Source: CAD feature listing. Evaluate the final solid. Frame: model axes, mm. Face numbers are marked on the shaded views. A direction names the side the tool comes from. Give positions to 0.01 mm unless a question says otherwise; leave off trailing zeros. Order: outer loops, then holes, each group sorted by start corner. A loop starts at its lowest first (then second) coordinate and runs counter-clockwise, first axis right, second up. Notation, with made-up numbers: M 74.5,33 L 114.5,33 A20 cw 114.5,51 Z; hole C -8,59.25 d11. An arc over 180 degrees is marked long. Use CSV: the item, a comma, the result in double quotes. Start each with the question number.
1. Section query C-C, the plane z = 0. Return the cut outline in (x, y).
2. Section query D-D, the plane x = 27. Return the cut outline in (y, z), plus the area to 3 significant figures.
3. Line query: line 1 along Z through (x, y) = (40.5, 3.55); line 2 along Z through (x, y) = (38, 4.5); line 3 along X through (y, z) = (1.75, -10). Output: solid intervals per line, ascending. Write a range as [from, to].
4. Section query A-A, the plane y = 2.7. Return the cut outline in (x, z), plus the area to 3 significant figures.
5. Pin query (flat end, axial travel): P1, Ø1.5, axis at x = 35, y = 5, coming from the -Z side; P2, Ø0.5, axis at y = 5.5, z = -7, coming from the +X side; P3, Ø10, axis at x = 12, z = -2, coming from the -Y side. Return the tip coordinate at first contact, or that it passes through.
6. Section query B-B, the plane x = 40.5. Return the cut outline in (y, z).
7. Mould query, pull axis X, two halves, no side actions, for the marked faces 1, 2, 3 and 4. Classes: released by +X, released by -X, zero draft, split by the parting line, or undercut.
8. Reachability of the marked faces 5, 6 and 7 from +Z, -Z, +X, -X, +Y, -Y: full face, straight path, thin tool, end or side. Return the list, or none.
from build123d import *

# Parameters (mm, degrees)
CROQUIS1_R              = 2.25
SALIENTE_EXTRUIR2_DEPTH = 6
CROQUIS2_W              = 8
CROQUIS2_H              = 30
CORTAR_EXTRUIR1_DEPTH   = 1


with BuildPart() as part:
    # Croquis1 → Saliente-Extruir2 (new body)
    with BuildSketch(Plane(origin=(0, 0, 0), x_dir=(1, 0, 0), z_dir=(0, 1, 0))):
        with BuildLine():
            Line((1, 20), (25.839745962, 20))
            Line((25.839745962, 20), (34.5, 15))
            Line((34.5, 15), (44.5, 15))
            Line((44.5, 15), (44.5, -15))
            Line((44.5, -15), (34.5, -15))
            Line((34.5, -15), (25.839745962, -20))
            Line((25.839745962, -20), (1, -20))
            Line((1, -20), (1, -16.720122607))
            ThreePointArc((1, -16.720122607), (16.75, 0), (1, 16.720122607))
            Line((1, 16.720122607), (1, 20))
        make_face()
        with Locations(Location((40.5, 10, 0), (0, 0, 270))):
            Circle(CROQUIS1_R, mode=Mode.SUBTRACT)
        with Locations(Location((40.5, -10, 0), (0, 0, 270))):
            Circle(CROQUIS1_R, mode=Mode.SUBTRACT)
    extrude(amount=SALIENTE_EXTRUIR2_DEPTH)

    # Croquis2 → Cortar-Extruir1 (cut)
    with BuildSketch(Plane(origin=(0, 6, 0), x_dir=(1, 0, 0), z_dir=(0, 1, 0))):
        with Locations((40.5, 0)):
            Rectangle(CROQUIS2_W, CROQUIS2_H)
    extrude(amount=-CORTAR_EXTRUIR1_DEPTH, mode=Mode.SUBTRACT)

    # Croquis3 → Cortar-Revolución1 (revolve, cut)
    with BuildSketch(Plane.XY):
        Polygon((16.75, 0), (16.75, 2), (17.904700538, 0), align=None)
    revolve(axis=Axis((0, 6, 0), (0, -1, 0)), mode=Mode.SUBTRACT)


solid = part.part
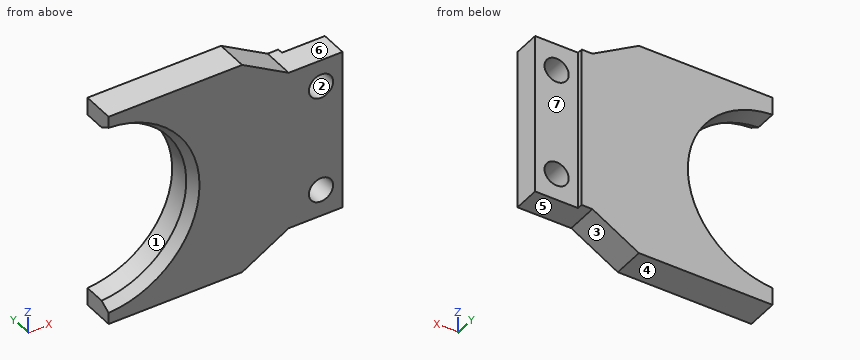
Result set:
1,outline,"M 16.75,2 L 17.9,0 L 44.5,0 L 44.5,5 L 36.5,5 L 36.5,6 L 16.75,6 Z"
2,outline,"M 0,-19.33 L 6,-19.33 L 6,19.33 L 0,19.33 Z"
2,area,"232 mm2"
3,line 1,"[-15, -12.25], [-7.75, 7.75], [12.25, 15]"
3,line 2,"[-15, 15]"
3,line 3,"[13.62, 38.25], [42.75, 44.5]"
4,outline,"M 1,-20 L 25.84,-20 L 34.5,-15 L 44.5,-15 L 44.5,15 L 34.5,15 L 25.84,20 L 1,20 L 1,16.72 A16.75 cw 1,-16.72 Z; hole C 40.5,-10 d4.5; hole C 40.5,10 d4.5"
4,area,"1,160 mm2"
5,P1,"z = -15.14"
5,P2,"x = 36.5"
5,P3,"y = 1.28"
6,outline,"M 0,-15 L 5,-15 L 5,-12.25 L 0,-12.25 Z; M 0,-7.75 L 5,-7.75 L 5,7.75 L 0,7.75 Z; M 0,12.25 L 5,12.25 L 5,15 L 0,15 Z"
7,face 1,"released by -X"
7,face 2,"undercut"
7,face 3,"released by +X"
7,face 4,"zero draft"
8,face 5,"-Z, +X, +Y, -Y"
8,face 6,"+Z, +X, +Y, -Y"
8,face 7,"+Z, -Z, +X, +Y"
